Could you check a few things on this drawing? It's one solid part, dimensions in mm from its lowest x, y, z. A direction names the side the tool comes from. Give positions to 0.01 mm unless a question says otherwise; leave off trailing zeros. Order: outer loops, then holes, each group sorted by start corner. A loop starts at its lowest first (then second) coordinate and runs counter-clockwise, first axis right, second up.
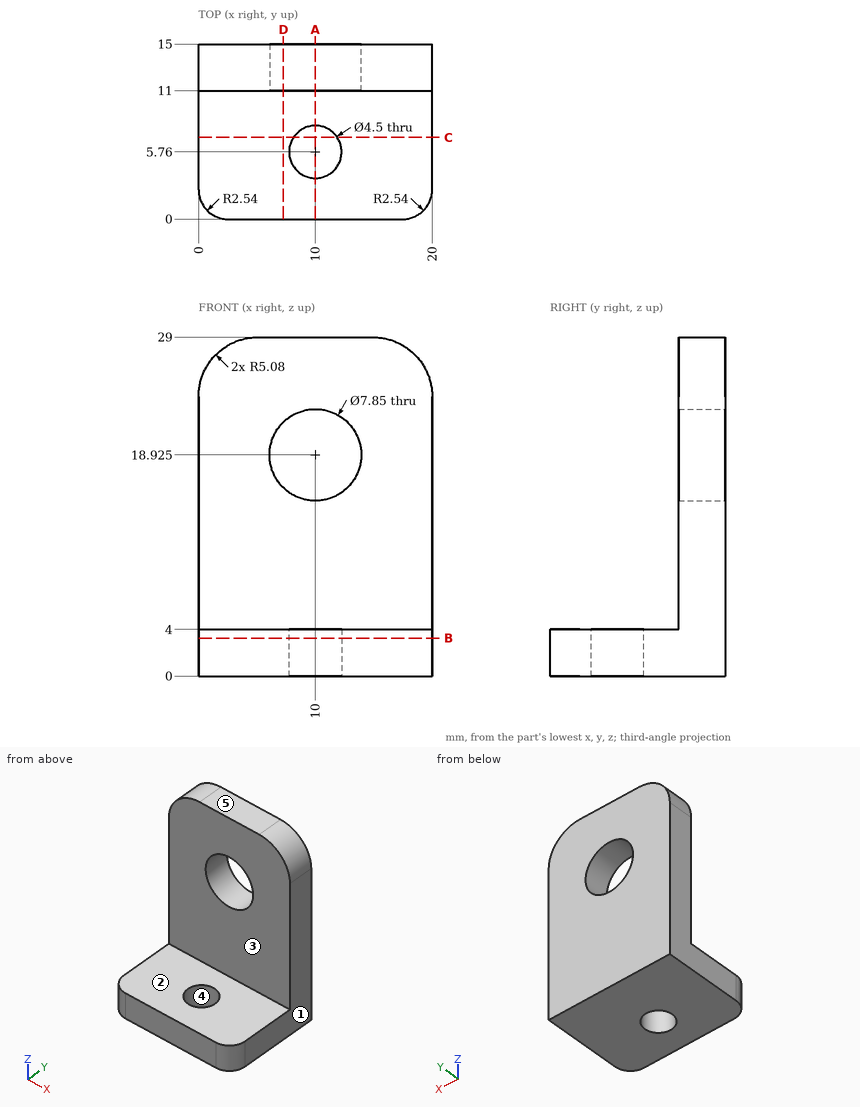
Item 1: Imagine slicing it at A-A on x = 10. List the corners of the cut face in (y, z) for me.
Findings:
outline: (0, 0) - (3.51, 0) - (3.51, 4) - (0, 4) - close; (8.01, 0) - (15, 0) - (15, 15) - (11, 15) - (11, 4) - (8.01, 4) - close; (11, 22.85) - (15, 22.85) - (15, 29) - (11, 29) - close
Item 2: We'd pull the mould along Y, two halves only. Please class the marked faces 3, 4 and 5: +Y half, -Y half, draft (parallel to the pull), parting line (faces both ways), or undercut.
Findings:
face 3: -Y half
face 4: undercut
face 5: draft
Item 3: Imagine slicing it at C-C on y = 7. List the corners of the cut face in (x, z) for me, then the cut area to 3 significant figures.
Findings:
outline: (0, 0) - (8.12, 0) - (8.12, 4) - (0, 4) - close; (11.88, 0) - (20, 0) - (20, 4) - (11.88, 4) - close
area: 65.0 mm2
Item 4: Imagine slicing it at D-D on x = 7.25. List the corners of the cut face in (y, z) for me, then the cut area to 3 significant figures.
Findings:
outline: (0, 0) - (15, 0) - (15, 16.12) - (11, 16.12) - (11, 4) - (0, 4) - close; (11, 21.73) - (15, 21.73) - (15, 29) - (11, 29) - close
area: 138 mm2
Item 5: Please list where these lines run through material, in increasing order: line 1 along Z through (x, y) = (10, 13.2); line 2 along Y through (x, z) = (10, 2.55); line 3 along Y through (x, z) = (8.25, 5.5).
Findings:
line 1: z = 0 to 15, 22.85 to 29
line 2: y = 0 to 3.51, 8.01 to 15
line 3: y = 11 to 15
Item 6: For pin 1 (6 mm diameter, centred on x = 3, z = 8.5, fed in from -Y); pin 2 (1 mm diameter, centred on y = 13, z = 26, fed in from -X), each with a flat end and sliding along its axis, tell me the tip position at first contact or that it passes through.
Findings:
pin 1: stops at y = 11
pin 2: stops at x = 0.25
Item 7: For the marked faces 1 and 2, which set-ups out of +Z, -Z, +X, -X, +Y, -Y let a thin tool reach every point of the face, with its end or its side?
Findings:
face 1: +Z, -Z, +X, +Y, -Y
face 2: +Z, +X, -X, -Y
Item 8: Imagine slicing it at B-B on z = 3.25. List the corners of the cut face in (x, y) for me.
Findings:
outline: (0, 2.54) arc R2.54 ccw to (2.54, 0) - (17.46, 0) arc R2.54 ccw to (20, 2.54) - (20, 15) - (0, 15) - close; hole circle Ø4.5 at (10, 5.76)
